Here's how the part is built. I have some questions about the finished solid (model axes, mm). A direction names the side the tool comes from. Give positions to 0.01 mm unless a question says otherwise; leave off trailing zeros. Write each loop counter-clockwise with the first axis right and the second up, starting at its lowest first coordinate (ties: lowest second). Pieces come first, ordered by that corner, then holes. Notation, with made-up numbers: (47.25, 41.5) -> (74.25, 41.5) arc R17 cw to (74.25, 62.5) -> close; hole circle Ø9 at (-6.75, -3). An arc over 180 degrees is marked (long way). Return JSON: item names as keys, results as strings.
from build123d import *

# Parameters (mm, degrees)
SALIENTE_EXTRUIR1_REACH             = 1008.239
SALIENTE_EXTRUIR1_DIRECTION_2_REACH = 1008.239


with BuildPart() as part:
    # Croquis2 → Revolución1 (revolve)
    with BuildSketch(Plane.XY, mode=Mode.PRIVATE) as revoluci_n1_sk:
        Polygon((-572.221380866, 0), (-290, 236.811856595), (-290, 243.338893041), (-580, 0), align=None)
        Polygon((-290, 799.338893041), (-580, 1042.677786083), (-572.221380866, 1042.677786083), (-290, 805.865929488), align=None)
    revolve(revoluci_n1_sk.sketch.rotate(Axis((0, 243.338893041, 0), (0, 1, 0)), 180), axis=Axis((0, 243.338893041, 0), (0, 1, 0)))

    # Saliente-Extruir1: up to this cone (the profile starts outside it)
    saliente_extruir1_end = Plane(origin=(0, 459.825, 0), z_dir=(0, 1, 0)).offset(96.175001) * Cone(1.192e-06, 1087.551425472, 912.563999, align=(Align.CENTER, Align.CENTER, Align.MIN), mode=Mode.PRIVATE)
    # Croquis3 → Saliente-Extruir1 (add, up to the surface)
    with BuildSketch(Plane(origin=(0, 459.825, 0), x_dir=(1, 0, 0), z_dir=(0, 1, 0)), mode=Mode.PRIVATE) as saliente_extruir1_sk1:
        Polygon((-562.011449548, 143.32875), (-188.170333372, 220.662469937), (-187.562612401, 217.724668851), (-561.403728577, 140.390948914), align=None)
    saliente_extruir1_tool1 = extrude(saliente_extruir1_sk1.sketch, amount=SALIENTE_EXTRUIR1_REACH, mode=Mode.PRIVATE) - saliente_extruir1_end
    add(saliente_extruir1_tool1.solids().sort_by_distance((-374.787031, 459.825, -180.526709))[0])
    # Croquis3 → Saliente-Extruir1 (add, up to the surface)
    with BuildSketch(Plane(origin=(0, 459.825, 0), x_dir=(1, 0, 0), z_dir=(0, 1, 0)), mode=Mode.PRIVATE) as saliente_extruir1_sk2:
        Polygon((-562.011449548, -143.32875), (-288.082841539, 33.290785673), (-286.457166797, 30.76944047), (-560.385774807, -145.850095203), align=None)
    saliente_extruir1_tool2 = extrude(saliente_extruir1_sk2.sketch, amount=SALIENTE_EXTRUIR1_REACH, mode=Mode.PRIVATE) - saliente_extruir1_end
    add(saliente_extruir1_tool2.solids().sort_by_distance((-424.234308, 459.825, 56.279655))[0])
    # Croquis3 → Saliente-Extruir1 (add, up to the surface)
    with BuildSketch(Plane(origin=(0, 459.825, 0), x_dir=(1, 0, 0), z_dir=(0, 1, 0)), mode=Mode.PRIVATE) as saliente_extruir1_sk3:
        Polygon((151.714649086, 247.149074958), (149.108430327, 245.663267507), (-39.963566042, 577.309863406), (-37.357347284, 578.795670858), align=None)
    saliente_extruir1_tool3 = extrude(saliente_extruir1_sk3.sketch, amount=SALIENTE_EXTRUIR1_REACH, mode=Mode.PRIVATE) - saliente_extruir1_end
    add(saliente_extruir1_tool3.solids().sort_by_distance((55.875542, 459.825, -412.229469))[0])
    # Croquis3 → Saliente-Extruir1 (add, up to the surface)
    with BuildSketch(Plane(origin=(0, 459.825, 0), x_dir=(1, 0, 0), z_dir=(0, 1, 0)), mode=Mode.PRIVATE) as saliente_extruir1_sk4:
        Polygon((-309.984830604, 490.213631793), (-57.361075176, 284.270482208), (-59.256655839, 281.945235135), (-311.880411267, 487.88838472), align=None)
    saliente_extruir1_tool4 = extrude(saliente_extruir1_sk4.sketch, amount=SALIENTE_EXTRUIR1_REACH, mode=Mode.PRIVATE) - saliente_extruir1_end
    add(saliente_extruir1_tool4.solids().sort_by_distance((-184.620743, 459.825, -386.079433))[0])
    # Croquis3 → Saliente-Extruir1 (add, up to the surface)
    with BuildSketch(Plane(origin=(0, 459.825, 0), x_dir=(1, 0, 0), z_dir=(0, 1, 0)), mode=Mode.PRIVATE) as saliente_extruir1_sk5:
        Polygon((281.935143099, -67.915941324), (279.716690352, -65.896419744), (536.704886451, 216.406168711), (538.923339197, 214.386647132), align=None)
    saliente_extruir1_tool5 = extrude(saliente_extruir1_sk5.sketch, amount=SALIENTE_EXTRUIR1_REACH, mode=Mode.PRIVATE) - saliente_extruir1_end
    add(saliente_extruir1_tool5.solids().sort_by_distance((409.320015, 459.825, -74.245114))[0])
    # Croquis3 → Saliente-Extruir1 (add, up to the surface)
    with BuildSketch(Plane(origin=(0, 459.825, 0), x_dir=(1, 0, 0), z_dir=(0, 1, 0)), mode=Mode.PRIVATE) as saliente_extruir1_sk6:
        Polygon((370.430288238, 446.297436197), (252.631747449, 142.398034329), (249.834539429, 143.482297809), (367.633080219, 447.381699677), align=None)
    saliente_extruir1_tool6 = extrude(saliente_extruir1_sk6.sketch, amount=SALIENTE_EXTRUIR1_REACH, mode=Mode.PRIVATE) - saliente_extruir1_end
    add(saliente_extruir1_tool6.solids().sort_by_distance((310.132414, 459.825, -294.889867))[0])
    # Croquis3 → Saliente-Extruir1 (add, up to the surface)
    with BuildSketch(Plane(origin=(0, 459.825, 0), x_dir=(1, 0, 0), z_dir=(0, 1, 0)), mode=Mode.PRIVATE) as saliente_extruir1_sk7:
        Polygon((22.530851972, -289.123435075), (23.765991531, -286.389494645), (371.665427797, -443.563495767), (370.430288238, -446.297436197), align=None)
    saliente_extruir1_tool7 = extrude(saliente_extruir1_sk7.sketch, amount=SALIENTE_EXTRUIR1_REACH, mode=Mode.PRIVATE) - saliente_extruir1_end
    add(saliente_extruir1_tool7.solids().sort_by_distance((197.09814, 459.825, 366.343465))[0])
    # Croquis3 → Saliente-Extruir1 (add, up to the surface)
    with BuildSketch(Plane(origin=(0, 459.825, 0), x_dir=(1, 0, 0), z_dir=(0, 1, 0)), mode=Mode.PRIVATE) as saliente_extruir1_sk8:
        Polygon((538.923339197, -214.386647132), (213.496081737, -196.263657061), (213.66289277, -193.268298305), (539.09015023, -211.391288375), align=None)
    saliente_extruir1_tool8 = extrude(saliente_extruir1_sk8.sketch, amount=SALIENTE_EXTRUIR1_REACH, mode=Mode.PRIVATE) - saliente_extruir1_end
    add(saliente_extruir1_tool8.solids().sort_by_distance((376.293116, 459.825, 203.827473))[0])
    # Croquis3 → Saliente-Extruir1 (add, up to the surface)
    with BuildSketch(Plane(origin=(0, 459.825, 0), x_dir=(1, 0, 0), z_dir=(0, 1, 0)), mode=Mode.PRIVATE) as saliente_extruir1_sk9:
        Polygon((-268.010310784, -110.772168496), (-265.02849981, -111.102021968), (-307.003019629, -490.543485264), (-309.984830604, -490.213631793), align=None)
    saliente_extruir1_tool9 = extrude(saliente_extruir1_sk9.sketch, amount=SALIENTE_EXTRUIR1_REACH, mode=Mode.PRIVATE) - saliente_extruir1_end
    add(saliente_extruir1_tool9.solids().sort_by_distance((-287.506665, 459.825, 300.657827))[0])
    # Croquis3 → Saliente-Extruir1 (add, up to the surface)
    with BuildSketch(Plane(origin=(0, 459.825, 0), x_dir=(1, 0, 0), z_dir=(0, 1, 0)), mode=Mode.PRIVATE) as saliente_extruir1_sk10:
        Polygon((-37.357347284, -578.795670858), (-120.683912471, -263.695645149), (-117.783609563, -262.928675109), (-34.457044376, -578.028700818), align=None)
    saliente_extruir1_tool10 = extrude(saliente_extruir1_sk10.sketch, amount=SALIENTE_EXTRUIR1_REACH, mode=Mode.PRIVATE) - saliente_extruir1_end
    add(saliente_extruir1_tool10.solids().sort_by_distance((-77.570478, 459.825, 420.862173))[0])

    # Saliente-Extruir1 direction 2: up to this cone (the profile starts outside it)
    saliente_extruir1_direction_2_end = Plane(origin=(0, 459.825, 0), z_dir=(0, -1, 0)).offset(-26.852785083) * Cone(1.192e-06, 1272.308615927, 1067.593689368, align=(Align.CENTER, Align.CENTER, Align.MIN), mode=Mode.PRIVATE)
    # Croquis3 → Saliente-Extruir1 direction 2 (add, up to the surface)
    with BuildSketch(Plane(origin=(0, 459.825, 0), x_dir=(1, 0, 0), z_dir=(0, 1, 0)), mode=Mode.PRIVATE) as saliente_extruir1_direction_2_sk1:
        Polygon((-562.011449548, 143.32875), (-188.170333372, 220.662469937), (-187.562612401, 217.724668851), (-561.403728577, 140.390948914), align=None)
    saliente_extruir1_direction_2_tool1 = extrude(saliente_extruir1_direction_2_sk1.sketch, amount=-SALIENTE_EXTRUIR1_DIRECTION_2_REACH, mode=Mode.PRIVATE) - saliente_extruir1_direction_2_end
    add(saliente_extruir1_direction_2_tool1.solids().sort_by_distance((-374.787031, 459.825, -180.526709))[0])
    # Croquis3 → Saliente-Extruir1 direction 2 (add, up to the surface)
    with BuildSketch(Plane(origin=(0, 459.825, 0), x_dir=(1, 0, 0), z_dir=(0, 1, 0)), mode=Mode.PRIVATE) as saliente_extruir1_direction_2_sk2:
        Polygon((-562.011449548, -143.32875), (-288.082841539, 33.290785673), (-286.457166797, 30.76944047), (-560.385774807, -145.850095203), align=None)
    saliente_extruir1_direction_2_tool2 = extrude(saliente_extruir1_direction_2_sk2.sketch, amount=-SALIENTE_EXTRUIR1_DIRECTION_2_REACH, mode=Mode.PRIVATE) - saliente_extruir1_direction_2_end
    add(saliente_extruir1_direction_2_tool2.solids().sort_by_distance((-424.234308, 459.825, 56.279655))[0])
    # Croquis3 → Saliente-Extruir1 direction 2 (add, up to the surface)
    with BuildSketch(Plane(origin=(0, 459.825, 0), x_dir=(1, 0, 0), z_dir=(0, 1, 0)), mode=Mode.PRIVATE) as saliente_extruir1_direction_2_sk3:
        Polygon((151.714649086, 247.149074958), (149.108430327, 245.663267507), (-39.963566042, 577.309863406), (-37.357347284, 578.795670858), align=None)
    saliente_extruir1_direction_2_tool3 = extrude(saliente_extruir1_direction_2_sk3.sketch, amount=-SALIENTE_EXTRUIR1_DIRECTION_2_REACH, mode=Mode.PRIVATE) - saliente_extruir1_direction_2_end
    add(saliente_extruir1_direction_2_tool3.solids().sort_by_distance((55.875542, 459.825, -412.229469))[0])
    # Croquis3 → Saliente-Extruir1 direction 2 (add, up to the surface)
    with BuildSketch(Plane(origin=(0, 459.825, 0), x_dir=(1, 0, 0), z_dir=(0, 1, 0)), mode=Mode.PRIVATE) as saliente_extruir1_direction_2_sk4:
        Polygon((-309.984830604, 490.213631793), (-57.361075176, 284.270482208), (-59.256655839, 281.945235135), (-311.880411267, 487.88838472), align=None)
    saliente_extruir1_direction_2_tool4 = extrude(saliente_extruir1_direction_2_sk4.sketch, amount=-SALIENTE_EXTRUIR1_DIRECTION_2_REACH, mode=Mode.PRIVATE) - saliente_extruir1_direction_2_end
    add(saliente_extruir1_direction_2_tool4.solids().sort_by_distance((-184.620743, 459.825, -386.079433))[0])
    # Croquis3 → Saliente-Extruir1 direction 2 (add, up to the surface)
    with BuildSketch(Plane(origin=(0, 459.825, 0), x_dir=(1, 0, 0), z_dir=(0, 1, 0)), mode=Mode.PRIVATE) as saliente_extruir1_direction_2_sk5:
        Polygon((281.935143099, -67.915941324), (279.716690352, -65.896419744), (536.704886451, 216.406168711), (538.923339197, 214.386647132), align=None)
    saliente_extruir1_direction_2_tool5 = extrude(saliente_extruir1_direction_2_sk5.sketch, amount=-SALIENTE_EXTRUIR1_DIRECTION_2_REACH, mode=Mode.PRIVATE) - saliente_extruir1_direction_2_end
    add(saliente_extruir1_direction_2_tool5.solids().sort_by_distance((409.320015, 459.825, -74.245114))[0])
    # Croquis3 → Saliente-Extruir1 direction 2 (add, up to the surface)
    with BuildSketch(Plane(origin=(0, 459.825, 0), x_dir=(1, 0, 0), z_dir=(0, 1, 0)), mode=Mode.PRIVATE) as saliente_extruir1_direction_2_sk6:
        Polygon((370.430288238, 446.297436197), (252.631747449, 142.398034329), (249.834539429, 143.482297809), (367.633080219, 447.381699677), align=None)
    saliente_extruir1_direction_2_tool6 = extrude(saliente_extruir1_direction_2_sk6.sketch, amount=-SALIENTE_EXTRUIR1_DIRECTION_2_REACH, mode=Mode.PRIVATE) - saliente_extruir1_direction_2_end
    add(saliente_extruir1_direction_2_tool6.solids().sort_by_distance((310.132414, 459.825, -294.889867))[0])
    # Croquis3 → Saliente-Extruir1 direction 2 (add, up to the surface)
    with BuildSketch(Plane(origin=(0, 459.825, 0), x_dir=(1, 0, 0), z_dir=(0, 1, 0)), mode=Mode.PRIVATE) as saliente_extruir1_direction_2_sk7:
        Polygon((22.530851972, -289.123435075), (23.765991531, -286.389494645), (371.665427797, -443.563495767), (370.430288238, -446.297436197), align=None)
    saliente_extruir1_direction_2_tool7 = extrude(saliente_extruir1_direction_2_sk7.sketch, amount=-SALIENTE_EXTRUIR1_DIRECTION_2_REACH, mode=Mode.PRIVATE) - saliente_extruir1_direction_2_end
    add(saliente_extruir1_direction_2_tool7.solids().sort_by_distance((197.09814, 459.825, 366.343465))[0])
    # Croquis3 → Saliente-Extruir1 direction 2 (add, up to the surface)
    with BuildSketch(Plane(origin=(0, 459.825, 0), x_dir=(1, 0, 0), z_dir=(0, 1, 0)), mode=Mode.PRIVATE) as saliente_extruir1_direction_2_sk8:
        Polygon((538.923339197, -214.386647132), (213.496081737, -196.263657061), (213.66289277, -193.268298305), (539.09015023, -211.391288375), align=None)
    saliente_extruir1_direction_2_tool8 = extrude(saliente_extruir1_direction_2_sk8.sketch, amount=-SALIENTE_EXTRUIR1_DIRECTION_2_REACH, mode=Mode.PRIVATE) - saliente_extruir1_direction_2_end
    add(saliente_extruir1_direction_2_tool8.solids().sort_by_distance((376.293116, 459.825, 203.827473))[0])
    # Croquis3 → Saliente-Extruir1 direction 2 (add, up to the surface)
    with BuildSketch(Plane(origin=(0, 459.825, 0), x_dir=(1, 0, 0), z_dir=(0, 1, 0)), mode=Mode.PRIVATE) as saliente_extruir1_direction_2_sk9:
        Polygon((-268.010310784, -110.772168496), (-265.02849981, -111.102021968), (-307.003019629, -490.543485264), (-309.984830604, -490.213631793), align=None)
    saliente_extruir1_direction_2_tool9 = extrude(saliente_extruir1_direction_2_sk9.sketch, amount=-SALIENTE_EXTRUIR1_DIRECTION_2_REACH, mode=Mode.PRIVATE) - saliente_extruir1_direction_2_end
    add(saliente_extruir1_direction_2_tool9.solids().sort_by_distance((-287.506665, 459.825, 300.657827))[0])
    # Croquis3 → Saliente-Extruir1 direction 2 (add, up to the surface)
    with BuildSketch(Plane(origin=(0, 459.825, 0), x_dir=(1, 0, 0), z_dir=(0, 1, 0)), mode=Mode.PRIVATE) as saliente_extruir1_direction_2_sk10:
        Polygon((-37.357347284, -578.795670858), (-120.683912471, -263.695645149), (-117.783609563, -262.928675109), (-34.457044376, -578.028700818), align=None)
    saliente_extruir1_direction_2_tool10 = extrude(saliente_extruir1_direction_2_sk10.sketch, amount=-SALIENTE_EXTRUIR1_DIRECTION_2_REACH, mode=Mode.PRIVATE) - saliente_extruir1_direction_2_end
    add(saliente_extruir1_direction_2_tool10.solids().sort_by_distance((-77.570478, 459.825, 420.862173))[0])


solid = part.part
1. Which directions (+Z, -Z, +X, -X, +Y, -Y) give clear straight access to the entire face, cutting with the end or side of a thin tool? Please do faces 4 (the face through (-211.87, 528.63, -406.36)), 5 (the face through (233.94, 528.62, 381.34)), 6 (the face through (-429.72, 119.97, -79.59)), 7 (the face through (384, 0, 427)).
Taken from the geometry:
{"face 4": "-X", "face 5": "+X", "face 6": "none", "face 7": "+Z, -Z, +X, -X, -Y"}
2. Suppose I cut it at B-B, the plane x = 0. List the corners of the cut face in (y, z) for me, and give its area (3 significant figures).
Taken from the geometry:
{"outline": "(0, -580) -> (55.99, -513.27) -> (986.68, -513.27) -> (1042.68, -580) -> (1042.68, -572.22) -> (805.87, -290) -> (799.34, -290) -> (981.6, -507.21) -> (61.08, -507.21) -> (243.34, -290) -> (236.81, -290) -> (0, -572.22) -> close; (0, 572.22) -> (236.81, 290) -> (243.34, 290) -> (0, 580) -> close; (799.34, 290) -> (805.87, 290) -> (1042.68, 572.22) -> (1042.68, 580) -> close", "area": "13,100 mm²"}
3. For pin 1 Ø12 at (x, y) = (-376, 237.5) entering from -Z; pin 2 Ø4 at (x, y) = (234, 383.5) entering from -Z; pin 3 Ø1 at (x, y) = (-327, 202) entering from -Z, each with a flat end and sliding along its axis, tell me the tip position at first contact or that it passes through.
Taken from the geometry:
{"pin 1": "stops at z = -183.05", "pin 2": "stops at z = 194.29", "pin 3": "stops at z = -192.05"}
4. If I drill on line 1 (Z direction, x = 228, y = 199); line 2 (Z direction, x = 0, y = 241); line 3 (X direction, y = 927, z = 102), over which ranges is the centre line in solid material (lowest first)? Write a range as [from, to].
Taken from the geometry:
{"line 1": "z = [-256.04, -245.53], [245.53, 256.04], [378.66, 381.95]", "line 2": "z = [-513.27, -507.21], [-292.79, -290], [290, 292.79]", "line 3": "x = [-497.91, -492.38], [-430.21, -422.22], [422.22, 430.21]"}
5. Suppose I cut it at C-C, the plane y = 398. Count the separate pieces of the cut face and the enclosed holes in it, and give its area (3 significant figures).
Taken from the geometry:
{"separate pieces": "10", "enclosed holes": "0", "area": "10,600 mm²"}
6. If we mould it in two halves opening along Z, with no side actions, what happens to faces 1 (the face through (237.571, 528.638, 386.274)), 2 (the face through (-185.441, 528.638, -388.684)), 3 (the face through (300.87, 922.71, 316.97))? For each: released by +Z, released by -Z, zero draft, split by the parting line, or undercut.
Taken from the geometry:
{"face 1": "released by +Z", "face 2": "released by -Z", "face 3": "undercut"}
7. Suppose I cut it at A-A, the plane z = 0. List the corners of the cut face in (x, y) for me.
Taken from the geometry:
{"outline": "(-580, 0) -> (-572.22, 0) -> (-290, 236.81) -> (-290, 243.34) -> (-334.18, 206.27) -> (-334.18, 836.41) -> (-290, 799.34) -> (-290, 805.87) -> (-572.22, 1042.68) -> (-580, 1042.68) -> (-339.72, 841.05) -> (-339.72, 201.62) -> close; (290, 236.81) -> (572.22, 0) -> (580, 0) -> (343.76, 198.23) -> (343.76, 844.45) -> (580, 1042.68) -> (572.22, 1042.68) -> (290, 805.87) -> (290, 799.34) -> (339.7, 841.05) -> (339.7, 201.63) -> (290, 243.34) -> close"}
